Study the drawing (mm; zero at the part's minimum x, y, z) and answer. Round coordinates to 2 decimals unless told otherwise and drop trailing zeros. Write each loop counter-clockwise with the first axis right and the second up, starting at its lowest first coordinate (ties: lowest second). Pieces come first, ordered by that corner, then holes.
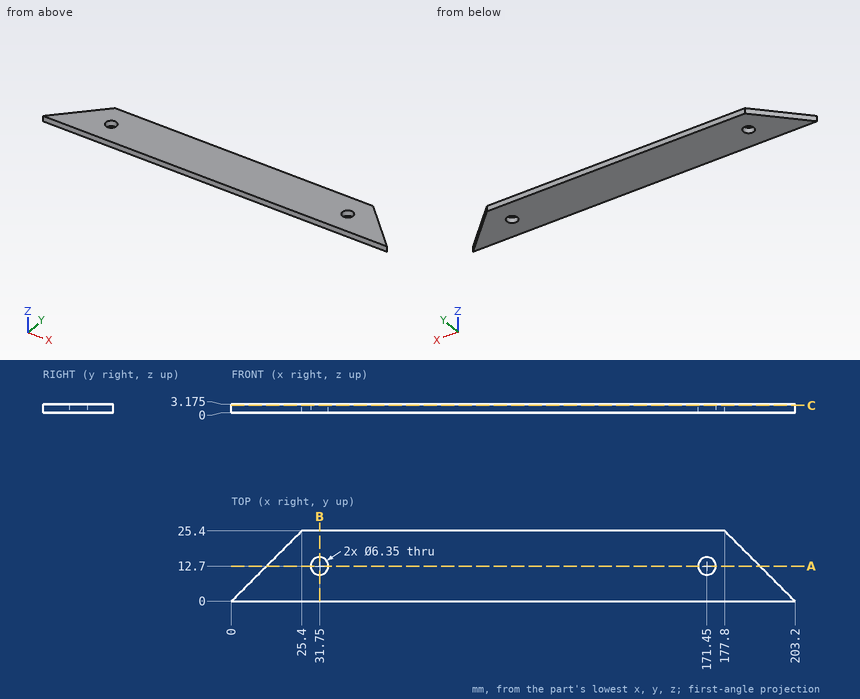
1. Section B-B on x = 31.75 is taken. Determine the outline of the cut face in (y, z) (3 decimals), plus the area to 3 significant figures.
Geometry says:
outline: (0, 0) - (9.525, 0) - (9.525, 3.175) - (0, 3.175) - close; (15.875, 0) - (25.4, 0) - (25.4, 3.175) - (15.875, 3.175) - close
area: 60.5 mm2
2. Straight lines are drawn through the part: line 1 along Y through (x, z) = (171.45, 0.7) (3 decimals); line 2 along Y through (x, z) = (30.5, 0.85); line 3 along X through (y, z) = (11, 1.35). For each, find the intervals that lie inside material, in ascending order.
Geometry says:
line 1: y = 0 to 9.525, 15.875 to 25.4
line 2: y = 0 to 9.78, 15.62 to 25.4
line 3: x = 11 to 29.07, 34.43 to 168.77, 174.13 to 192.2
3. Given pin 1 (4 mm diameter, centred on x = 171.45, y = 12.7, fed in from -Z), flat-ended and moving along its own axis, determine where the tip first touches the part or whether it passes through.
Geometry says:
pin 1: passes through
4. Section C-C on z = 2.65 is taken. Determine the outline of the cut face in (x, y) (3 decimals), plus the area to 3 significant figures.
Geometry says:
outline: (0, 0) - (203.2, 0) - (177.8, 25.4) - (25.4, 25.4) - close; hole circle Ø6.35 at (31.75, 12.7); hole circle Ø6.35 at (171.45, 12.7)
area: 4,450 mm2
5. Section A-A on y = 12.7 is taken. Determine the outline of the cut face in (x, z) (3 decimals), plus the area to 3 significant figures.
Geometry says:
outline: (12.7, 0) - (28.575, 0) - (28.575, 3.175) - (12.7, 3.175) - close; (34.925, 0) - (168.275, 0) - (168.275, 3.175) - (34.925, 3.175) - close; (174.625, 0) - (190.5, 0) - (190.5, 3.175) - (174.625, 3.175) - close
area: 524 mm2
